Geometry: final body of the model. Coordinates: model frame, mm. Face numbers are marked on the shaded views. A direction names the side the tool comes from. Round coordinates to 2 decimals unless told otherwise and drop trailing zeros. Loops run counter-clockwise (first coordinate to the right, second up) from the corner with the lowest first, then second, coordinate; pieces in that order, holes last. Notation, with made-up numbers: (23.25, -29) - (38.25, -29) arc R5 ccw to (38.25, -21) - close; hole circle Ø2 at (0, 16.25). An arc over 180 degrees is marked (long way). Use CSV: the item, a comma, the result in double quotes.
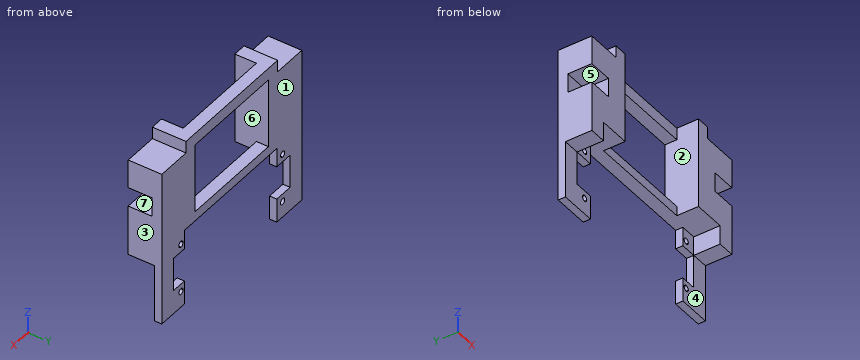
from build123d import *

# Parameters (mm, degrees)
SKETCH1_W           = 70
SKETCH1_H           = 30
SKETCH1_W_2         = 55
SKETCH1_H_2         = 5
BOSS_EXTRUDE1_DEPTH = 5
BOSS_EXTRUDE2_DEPTH = 9
CUT_EXTRUDE1_DEPTH  = 2
BOSS_EXTRUDE3_DEPTH = 3
SKETCH7_W           = 54
SKETCH7_H           = 2
SKETCH7_W_2         = 1.5
SKETCH7_H_2         = 8
CUT_EXTRUDE4_DEPTH  = 10
SKETCH8_W           = 10
SKETCH8_H           = 8
CUT_EXTRUDE5_DEPTH  = 10


with BuildPart() as part:
    # Sketch1 → Boss-Extrude1 (new body)
    with BuildSketch(Plane(origin=(0, 0, 0), x_dir=(1, 0, 0), z_dir=(0, 1, 0))):
        Polygon((-5.25, -11), (-29.5, -11), (-42, -11), (-42, -76), (-27.5, -76), (-22, -76), (-22, -47), (22, -47), (22, -76), (27.5, -76), (42, -76), (42, -11), (29.5, -11), (5.25, -11), align=None)
        with Locations((0, -28)):
            Rectangle(SKETCH1_W, SKETCH1_H, mode=Mode.SUBTRACT)
        Polygon((-5.25, -11), (-29.5, -11), (-42, -11), (-42, -76), (-27.5, -76), (-22, -76), (-22, -47), (22, -47), (22, -76), (27.5, -76), (42, -76), (42, -11), (29.5, -11), (5.25, -11), align=None)
        with Locations((0, -28)):
            Rectangle(SKETCH1_W, SKETCH1_H, mode=Mode.SUBTRACT)
        Polygon((-5.25, -11), (-29.5, -11), (-42, -11), (-42, -76), (-27.5, -76), (-22, -76), (-22, -47), (22, -47), (22, -76), (27.5, -76), (42, -76), (42, -11), (29.5, -11), (5.25, -11), align=None)
        with Locations((0, -28)):
            Rectangle(SKETCH1_W, SKETCH1_H, mode=Mode.SUBTRACT)
        with Locations((0, -78.5)):
            Rectangle(SKETCH1_W_2, SKETCH1_H_2)
    extrude(amount=BOSS_EXTRUDE1_DEPTH)

    # Sketch2 → Boss-Extrude2 (add)
    with BuildSketch(Plane.XZ):
        Polygon((-27.5, 76), (-42, 76), (-42, 35), (-35, 35), (-35, 43), (-22, 43), (-22, 81), (-27.5, 81), align=None)
        Polygon((22, 81), (22, 43), (35, 43), (35, 35), (42, 35), (42, 76), (27.5, 76), (27.5, 81), align=None)
    extrude(amount=BOSS_EXTRUDE2_DEPTH)

    # Sketch3 → Cut-Extrude1 (cut)
    with BuildSketch(Plane.XZ):
        Polygon((-42, 35), (-42, 11), (42, 11), (42, 35), (35, 35), (35, 13), (-35, 13), (-35, 35), align=None)
    extrude(amount=-CUT_EXTRUDE1_DEPTH, mode=Mode.SUBTRACT)

    # Sketch6 → Boss-Extrude3 (add)
    with BuildSketch(Plane(origin=(0, 5, 0), x_dir=(1, 0, 0), z_dir=(0, 1, 0))):
        with BuildLine():
            ThreePointArc((-30.5, -19), (-31.383883476, -16.866116524), (-29.25, -17.75))
            Line((-29.25, -17.75), (-27, -17.75))
            Line((-27, -17.75), (-27, -13))
            Line((-27, -13), (-35, -13))
            Line((-35, -13), (-35, -21))
            Line((-35, -21), (-30.5, -21))
            Line((-30.5, -21), (-30.5, -19))
        make_face()
        with BuildLine():
            Line((-27, -17.75), (-29.25, -17.75))
            ThreePointArc((-29.25, -17.75), (-29.616116524, -18.633883476), (-30.5, -19))
            Line((-30.5, -19), (-30.5, -21))
            Line((-30.5, -21), (-27, -21))
            Line((-27, -21), (-27, -17.75))
        make_face()
        with BuildLine():
            Line((-30.5, -37), (-30.5, -35))
            Line((-30.5, -35), (-35, -35))
            Line((-35, -35), (-35, -43))
            Line((-35, -43), (-27, -43))
            Line((-27, -43), (-27, -38.25))
            Line((-27, -38.25), (-29.25, -38.25))
            ThreePointArc((-29.25, -38.25), (-31.383883476, -39.133883476), (-30.5, -37))
        make_face()
        with BuildLine():
            Line((-27, -35), (-30.5, -35))
            Line((-30.5, -35), (-30.5, -37))
            ThreePointArc((-30.5, -37), (-29.616116524, -37.366116524), (-29.25, -38.25))
            Line((-29.25, -38.25), (-27, -38.25))
            Line((-27, -38.25), (-27, -35))
        make_face()
        with BuildLine():
            Line((35, -35), (30.5, -35))
            Line((30.5, -35), (30.5, -37))
            ThreePointArc((30.5, -37), (31.383883476, -37.366116524), (31.75, -38.25))
            ThreePointArc((31.75, -38.25), (30.5, -39.5), (29.25, -38.25))
            Line((29.25, -38.25), (27, -38.25))
            Line((27, -38.25), (27, -43))
            Line((27, -43), (35, -43))
            Line((35, -43), (35, -35))
        make_face()
        with BuildLine():
            Line((30.5, -37), (30.5, -35))
            Line((30.5, -35), (27, -35))
            Line((27, -35), (27, -38.25))
            Line((27, -38.25), (29.25, -38.25))
            ThreePointArc((29.25, -38.25), (29.616116524, -37.366116524), (30.5, -37))
        make_face()
        with BuildLine():
            Line((27, -13), (27, -17.75))
            Line((27, -17.75), (29.25, -17.75))
            ThreePointArc((29.25, -17.75), (30.5, -16.5), (31.75, -17.75))
            ThreePointArc((31.75, -17.75), (31.383883476, -18.633883476), (30.5, -19))
            Line((30.5, -19), (30.5, -21))
            Line((30.5, -21), (35, -21))
            Line((35, -21), (35, -13))
            Line((35, -13), (27, -13))
        make_face()
        with BuildLine():
            Line((29.25, -17.75), (27, -17.75))
            Line((27, -17.75), (27, -21))
            Line((27, -21), (30.5, -21))
            Line((30.5, -21), (30.5, -19))
            ThreePointArc((30.5, -19), (29.616116524, -18.633883476), (29.25, -17.75))
        make_face()
    extrude(amount=-BOSS_EXTRUDE3_DEPTH)

    # Sketch7 → Cut-Extrude4 (cut)
    with BuildSketch(Plane(origin=(0, 5, 0), x_dir=(1, 0, 0), z_dir=(0, 1, 0))):
        Polygon((27, -11), (27, -13), (27, -21), (28.5, -21), (28.5, -11), align=None)
        with Locations((0, -12)):
            Rectangle(SKETCH7_W, SKETCH7_H)
        with Locations((27.75, -39)):
            Rectangle(SKETCH7_W_2, SKETCH7_H_2)
    extrude(amount=-CUT_EXTRUDE4_DEPTH, mode=Mode.SUBTRACT)

    # Sketch8 → Cut-Extrude5 (cut)
    with BuildSketch(Plane.XZ.offset(9)):
        with Locations((-37, 60)):
            Rectangle(SKETCH8_W, SKETCH8_H)
        with Locations((37, 60)):
            Rectangle(SKETCH8_W, SKETCH8_H)
    extrude(amount=-CUT_EXTRUDE5_DEPTH, mode=Mode.SUBTRACT)


solid = part.part
Item 1: Reachability of the marked faces 4, 5, 6 and 7 from +Z, -Z, +X, -X, +Y, -Y: full face, straight path, thin tool, end or side. Return the list, or none.
Final values:
face 4,"-Z, +X, -X, -Y"
face 5,"-X, -Y"
face 6,"-Y"
face 7,"+X, -Y"
Item 2: Mould query, pull axis X, two halves, no side actions, for the marked faces 1, 2 and 3. Classes: released by +X, released by -X, zero draft, split by the parting line, or undercut.
Final values:
face 1,"zero draft"
face 2,"undercut"
face 3,"released by +X"
Item 3: Pin query (flat end, axial travel): P1, Ø12, axis at x = 8.5, z = 66.5, coming from the +Y side; P2, Ø0.9, axis at x = -29.5, y = 3.5, coming from the +Z side; P3, Ø9, axis at x = -30, z = 37.5, coming from the -Y side; P4, Ø2, axis at x = 40, y = -2, coming from the -Z side. Return the tip coordinate at first contact, or that it passes through.
Final values:
P1,"passes through"
P2,"stops at z = 76"
P3,"stops at y = 2"
P4,"stops at z = 35"
Item 4: Material intervals for line 1 (Z direction, x = -30.5, y = 3.15); line 2 (X direction, y = 4.45, z = 17.75); line 3 (X direction, y = -3, z = 62.5), sorted ascending.
Final values:
line 1,"z = 11 to 16.5, 19 to 21, 35 to 37, 39.5 to 76"
line 2,"x = -42 to -31.75, -29.25 to -27, 28.5 to 29.25, 31.75 to 42"
line 3,"x = -32 to -22, 22 to 32"
Item 5: Section B-B on y = -7.75. Return the cut outline in (x, z).
Final values:
outline,"(-42, 35) - (-35, 35) - (-35, 43) - (-22, 43) - (-22, 81) - (-27.5, 81) - (-27.5, 76) - (-42, 76) - (-42, 64) - (-32, 64) - (-32, 56) - (-42, 56) - close; (22, 43) - (35, 43) - (35, 35) - (42, 35) - (42, 56) - (32, 56) - (32, 64) - (42, 64) - (42, 76) - (27.5, 76) - (27.5, 81) - (22, 81) - close"
Item 6: Section A-A on z = 23. Return the cut outline in (x, y), plus the area to 3 significant figures.
Final values:
outline,"(-42, 2) - (-35, 2) - (-35, 5) - (-42, 5) - close; (35, 2) - (42, 2) - (42, 5) - (35, 5) - close"
area,"42.0 mm²"
Item 7: Section C-C on x = -14. Return the cut outline in (y, z), plus the area to 3 significant figures.
Final values:
outline,"(0, 43) - (5, 43) - (5, 47) - (0, 47) - close; (0, 76) - (5, 76) - (5, 81) - (0, 81) - close"
area,"45.0 mm²"
Item 8: Section D-D on x = -37. Return the cut outline in (y, z).
Final values:
outline,"(-9, 35) - (2, 35) - (2, 11) - (5, 11) - (5, 76) - (-9, 76) - (-9, 64) - (1, 64) - (1, 56) - (-9, 56) - close"
